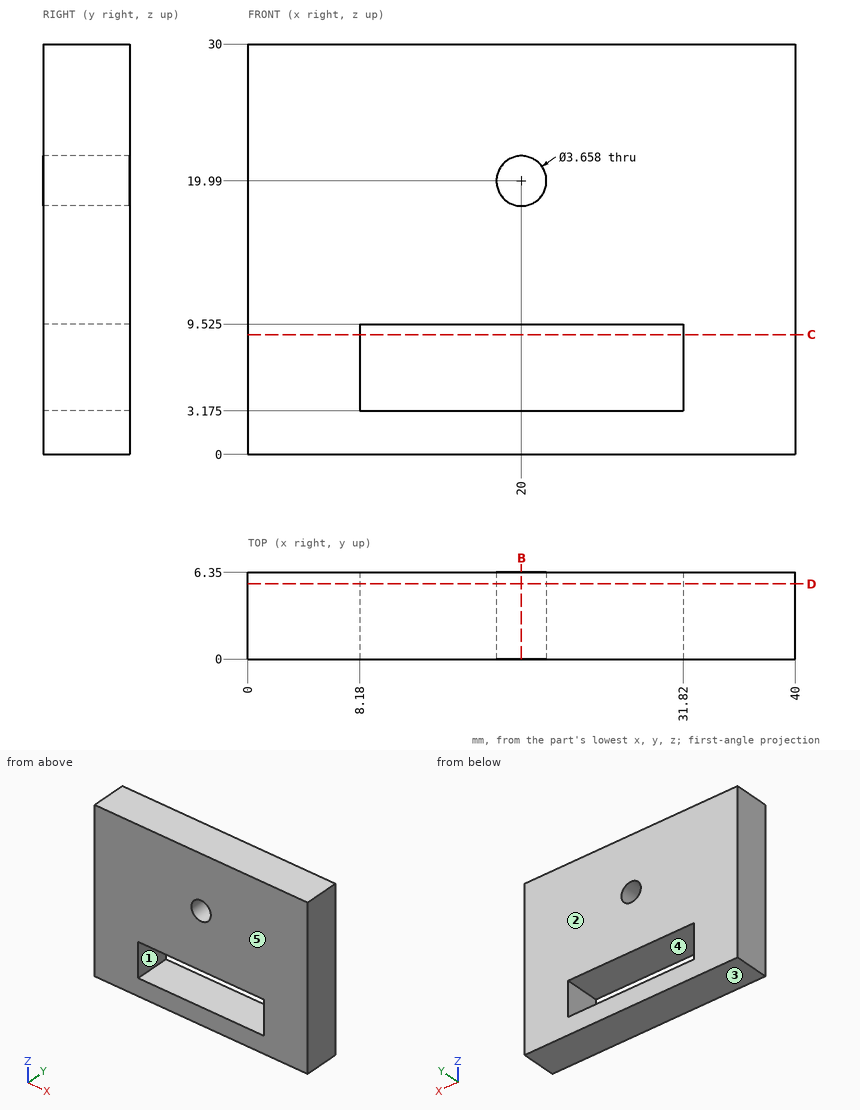
Can you work these out from the drawing? Everything is in mm from the part's minimum corner. A direction names the side the tool comes from. Round coordinates to 2 decimals unless told otherwise and drop trailing zeros. Write each loop counter-clockwise with the first axis right and the second up, starting at its lowest first coordinate (ties: lowest second). Pieces come first, ordered by that corner, then holes. Notation, with made-up numbers: M -13.5,32.25 L 43.5,32.25 A17 ccw 43.5,53.25 Z; hole C -8,-6.5 d2. An arc over 180 degrees is marked long. Use a Markdown table: item, result.
Item 1: We'd pull the mould along Z, two halves only. Please class the marked faces 1, 2 and 3: released by +Z, released by -Z, zero draft, split by the parting line, or undercut.
Found:
| item | result |
|---|---|
| face 1 | undercut |
| face 2 | zero draft |
| face 3 | released by -Z |
Item 2: I want a section at D-D (y = 5.5). List the corners of the cut face in (x, z) for me (1 decimal), and give its area (3 significant figures).
Found:
| item | result |
|---|---|
| outline | M 0,0 L 40,0 L 40,30 L 0,30 Z; hole M 8.2,3.2 L 31.8,3.2 L 31.8,9.5 L 8.2,9.5 Z; hole C 20,20 d3.7 |
| area | 1,040 mm2 |
Item 3: I want a section at B-B (x = 20). State how many separate pieces and enclosed holes the cut face has, and give its area (3 significant figures).
Found:
| item | result |
|---|---|
| separate pieces | 3 |
| enclosed holes | 0 |
| area | 127 mm2 |
Item 4: Which directions (+Z, -Z, +X, -X, +Y, -Y) give clear straight access to the entire face, cutting with the end or side of a thin tool? Please do the marked faces 4 and 5.
Found:
| item | result |
|---|---|
| face 4 | +Y, -Y |
| face 5 | +Z, -Z, +X, -X, -Y |
Item 5: I want a section at C-C (z = 8.75). List the corners of the cut face in (x, y) for me.
Found:
| item | result |
|---|---|
| outline | M 0,0 L 8.18,0 L 8.18,6.35 L 0,6.35 Z; M 31.82,0 L 40,0 L 40,6.35 L 31.82,6.35 Z |
Item 6: If I drill on line 1 along Z through (x, y) = (20, 1.5) (1 decimal); line 2 along Z through (x, y) = (26, 5.75) (1 decimal); line 3 along X through (y, z) = (5.5, 7.25), over which ranges is the centre line in solid material (lowest first)? Write a range as [from, to].
Found:
| item | result |
|---|---|
| line 1 | z = [0, 3.2], [9.5, 18.2], [21.8, 30] |
| line 2 | z = [0, 3.2], [9.5, 30] |
| line 3 | x = [0, 8.18], [31.82, 40] |
